Verification items for the finished model (mm, model axes). Face numbers are marked on the shaded views. A direction names the side the tool comes from. Coordinates: 2 decimals unless noted, no trailing zeros. Order: outer loops, then holes, each group sorted by start corner. A loop starts at its lowest first (then second) coordinate and runs counter-clockwise, first axis right, second up. Notation, with made-up numbers: M 49,23 L 57,23 A18 cw 57,49 Z; hole C 40.5,32 d2. An arc over 180 degrees is marked long. Return JSON: item names as keys, results as strings. Group by question number.
Q1. Mould release check, pull along Y, two halves, no side actions. Record for the marked faces 1, 2 and 3: pulls with the +Y half, pulls with the -Y half, needs draft (parallel to the pull), parting line crosses it, or undercut.
Q2. Access from +Z, -Z, +X, -X, +Y, -Y to the whole of each face (thin tool, end or side, straight path). Record for the marked faces 4 and 5.
Q3. Go/stop test with flat-tipped pins: pin 1 Ø3.5 at (y, z) = (6.59, 6) entering from +X; pin 2 Ø6 at (x, y) = (-2.5, -23.5) entering from +Z; pin 3 Ø5 at (y, z) = (7, 6) entering from -X. Record where each tip stops, or that it passes through.
Q4. Section check B-B, the plane x = 1.5. Enter the section's corners in (y, z), then the cut area to 3 significant figures.
Q5. Section check C-C, the plane y = -15. Enter the section's corners in (x, z), then the cut area to 3 significant figures.
Q6. Section check D-D, the plane y = 7.5. Enter the section's corners in (x, z).
Q7. Section check A-A, the plane x = -8. Enter the section's corners in (y, z), then the cut area to 3 significant figures.
Q8. Thickness scan on probe 1 along Y at (x, z) = (-8.55, 6); probe 2 along Z at (x, y) = (3.5, 0); probe 3 along X at (y, z) = (2, 8.75). Record the ranges inside material, lowest first.
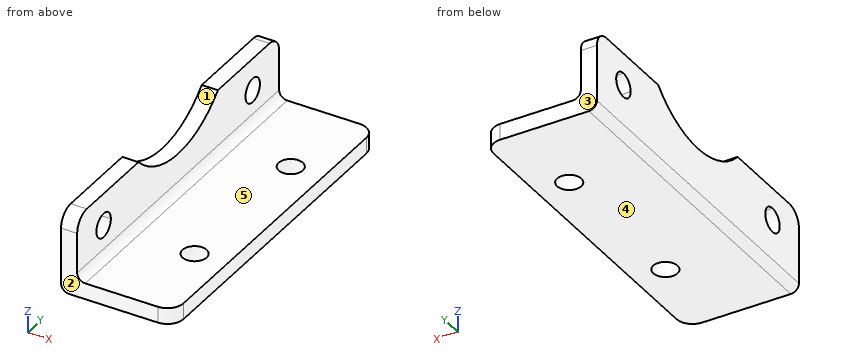
from build123d import *

# Parameters (mm, degrees)
SKETCH_1_W      = 14
SKETCH_1_H      = 42
SKETCH_1_R      = 1.5
EXTRUDE_1_DEPTH = 2
EXTRUDE_2_DEPTH = 2
FILLET_1_R      = 2
FILLET_2_R      = 1


with BuildPart() as part:
    # 草图1 → 凸台-拉伸1 (new body)
    with BuildSketch(Plane.XY):
        with Locations((-2.509513742, -8.913319239)):
            Rectangle(SKETCH_1_W, SKETCH_1_H)
        with Locations((0.490486258, 1.086680761)):
            Circle(SKETCH_1_R, mode=Mode.SUBTRACT)
        with Locations((0.490486258, -18.913319239)):
            Circle(SKETCH_1_R, mode=Mode.SUBTRACT)
    extrude(amount=EXTRUDE_1_DEPTH)

    # 草图2 → 凸台-拉伸2 (add)
    with BuildSketch(Plane.ZY.offset(9.509513742)):
        with BuildLine():
            Line((10, 12.086680761), (2, 12.086680761))
            Line((2, 12.086680761), (2, -29.913319239))
            Line((2, -29.913319239), (10, -29.913319239))
            Line((10, -29.913319239), (10, -17.17467506))
            ThreePointArc((10, -17.17467506), (6.5, -8.913319239), (10, -0.651963418))
            Line((10, -0.651963418), (10, 12.086680761))
        make_face()
        with BuildLine():
            ThreePointArc((7.5, -24.413319239), (4.939339828, -25.473979411), (6, -22.913319239))
            ThreePointArc((6, -22.913319239), (7.060660172, -23.352659067), (7.5, -24.413319239))
        make_face(mode=Mode.SUBTRACT)
        with BuildLine():
            ThreePointArc((7.5, 6.586680761), (7.060660172, 5.526020589), (6, 5.086680761))
            ThreePointArc((6, 5.086680761), (4.939339828, 7.647340933), (7.5, 6.586680761))
        make_face(mode=Mode.SUBTRACT)
    extrude(amount=-EXTRUDE_2_DEPTH)

    # 圆角1
    fillet_1_edges = [part.edges().sort_by_distance(p)[0] for p in [
        (4.490486258, -29.913319239, 1),
        (4.490486258, 12.086680761, 1),
        (-8.509513742, -29.913319239, 10),
        (-8.509513742, 12.086680761, 10),
    ]]
    fillet(fillet_1_edges, radius=FILLET_1_R)

    # 圆角2
    fillet_2_edges = [part.edges().sort_by_distance(p)[0] for p in [
        (-7.509513742, -8.913319239, 2),
        (-9.509513742, -8.913319239, 0),
    ]]
    fillet(fillet_2_edges, radius=FILLET_2_R)


solid = part.part
Numbers:
{
 "1": {"face 1": "undercut", "face 2": "pulls with the -Y half", "face 3": "pulls with the +Y half"},
 "2": {"face 4": "-Z, +X, -X, +Y, -Y", "face 5": "+Z, +X, +Y, -Y"},
 "3": {"pin 1": "stops at x = -7.51", "pin 2": "stops at z = 2", "pin 3": "stops at x = -9.51"},
 "4": {"outline": "M -29.91,0 L -20.02,0 L -20.02,2 L -29.91,2 Z; M -17.8,0 L -0.02,0 L -0.02,2 L -17.8,2 Z; M 2.2,0 L 12.09,0 L 12.09,2 L 2.2,2 Z", "area": "75.1 mm2"},
 "5": {"outline": "M -9.51,1 A1 ccw -8.51,0 L 4.49,0 L 4.49,2 L -6.51,2 A1 cw -7.51,3 L -7.51,8.24 L -9.51,8.24 Z", "area": "40.5 mm2"},
 "6": {"outline": "M -9.51,1 A1 ccw -8.51,0 L 4.49,0 L 4.49,2 L -6.51,2 A1 cw -7.51,3 L -7.51,4.81 L -9.51,4.81 Z; M -9.51,7.19 L -7.51,7.19 L -7.51,10 L -9.51,10 Z"},
 "7": {"outline": "M -29.91,0 L 12.09,0 L 12.09,8 A2 ccw 10.09,10 L -0.65,10 A11.5 cw -17.17,10 L -27.91,10 A2 ccw -29.91,8 Z; hole C -24.41,6 d3; hole C 6.59,6 d3", "area": "364 mm2"},
 "8": {"probe 1": "y = -29.91 to -25.91, -22.91 to 5.09, 8.09 to 12.09", "probe 2": "z = 0 to 2", "probe 3": "x = -9.51 to -7.51"}
}
